from build123d import *

# Parameters (mm, degrees)
F0_R     = 10
F1_DEPTH = 50
F0_W     = 50
F0_H     = 15
F2_DEPTH = 15
F3_W     = 50
F3_H     = 15
F4_DEPTH = 35
F6_DEPTH = 27.501
F8_DEPTH = 257.5


with BuildPart() as f1:
    # F0 (on Front) → F1 (new body)
    with BuildSketch(Plane.XZ):
        with BuildLine():
            ThreePointArc((18.540496, 7.5), (13.624005, 14.641943), (6.146908, 19.03196))
            ThreePointArc((6.146908, 19.03196), (-18.120519, -8.464442), (18.540496, -7.5))
            ThreePointArc((18.540496, -7.5), (19.631734, -3.820345), (20, 0))
            ThreePointArc((20, 0), (19.631734, 3.820345), (18.540496, 7.5))
        make_face()
        Circle(F0_R, mode=Mode.SUBTRACT)
        with BuildLine():
            Line((27.149505, -7.5), (27.149505, 7.5))
            Line((27.149505, 7.5), (18.540496, 7.5))
            ThreePointArc((18.540496, 7.5), (19.631734, 3.820345), (20, 0))
            ThreePointArc((20, 0), (19.631734, -3.820345), (18.540496, -7.5))
            Line((18.540496, -7.5), (27.149505, -7.5))
        make_face()
    extrude(amount=F1_DEPTH)

    # F0 (on Front) → F2 (join)
    with BuildSketch(Plane.XZ):
        with BuildLine():
            Line((77.149505, 7.5), (77.149505, 24.5))
            ThreePointArc((77.149505, 24.5), (61.595967, 43.999461), (39.126608, 33.170362))
            ThreePointArc((39.126608, 33.170362), (25.287149, 19.918772), (6.146908, 19.03196))
            ThreePointArc((6.146908, 19.03196), (13.624005, 14.641943), (18.540496, 7.5))
            Line((18.540496, 7.5), (27.149505, 7.5))
            Line((27.149505, 7.5), (77.149505, 7.5))
        make_face()
        with Locations((57.149505, 24.5)):
            Circle(F0_R, mode=Mode.SUBTRACT)
        with Locations((52.149505, 0)):
            Rectangle(F0_W, F0_H)
    extrude(amount=F2_DEPTH)

    # F3 (on face) → F4 (join)
    with BuildSketch(Plane.XZ.offset(15)):
        with Locations((52.149505, 0)):
            Rectangle(F3_W, F3_H)
    extrude(amount=F4_DEPTH)

    # F5 (on face) → F6 (join, through all)
    with BuildSketch(Plane.XY.offset(7.5)):
        Polygon((77.149505, -25), (27.149505, -50), (77.149505, -50), align=None)
    extrude(amount=-F6_DEPTH)

    # F7 (on face) → F8 (cut)
    with BuildSketch(Plane.XY.offset(7.5)):
        Polygon((77.149505, -25), (27.149505, -50), (77.149505, -50), align=None)
    extrude(amount=-F8_DEPTH, mode=Mode.SUBTRACT)


solid = f1.part
Can you work these out from the model? Positions are in its coordinate system, mm. A direction names the side the tool comes from. Coordinates: 2 decimals unless noted, no trailing zeros. Write each loop counter-clockwise with the first axis right and the second up, starting at its lowest first coordinate (ties: lowest second). Pieces come first, ordered by that corner, then holes. Notation, with made-up numbers: (3, -18.75) - (62, -18.75) arc R22 cw to (62, 16.25) - close; hole circle Ø8 at (-25, 31). An arc over 180 degrees is marked (long way). Return JSON: item names as keys, results as strings. Group by question number.
Item 1: I'm going to push flat-ended pins straight in: pin 1 Ø6 at (x, y) = (5.5, -26.5) entering from -Z; pin 2 Ø2 at (y, z) = (-17.5, 9) entering from +X; pin 3 Ø15 at (x, y) = (42, -23.5) entering from -Z. Where does each tip first touch, or does it pass through?
Item 2: We'd pull the mould along X, two halves only. Please class faces 4 (the face through (25.54, -7.4, 20.03)), 5 (the face through (8, -50, 9)), 6 (the face through (52.5, -37.325, 0.105)): pulls with the +X half, pulls with the -X half, needs draft (parallel to the pull), parting line crosses it, or undercut.
Item 3: If we section it at B-B (x = 0): Write out the boundary of the cut face in (y, z).
Item 4: Which directions (+Z, -Z, +X, -X, +Y, -Y) give clear straight access to the entire face, cutting with the end or side of a thin tool? Please do faces 1 (the face through (41, -19, -7.5)), 2 (the face through (49, -15, 18)), 3 (the face through (61.963, -7.395, 43.912)).
Item 5: If we section it at A-A (y = -13): Write out the boundary of the cut face in (x, z), then the cut area to 3 significant figures.
Item 6: If we section it at C-C (z = 0): Write out the boundary of the cut face in (x, y).
Item 7: If we section it at D-D (y = -18): Write out the boundary of the cut face in (x, z), then the cut area to 3 significant figures.
Item 8: Please list where these lines run through material, in increasing order: probe 1 along Z at (x, y) = (0, -19); probe 2 along Y at (x, z) = (50.5, 40); probe 3 along Z at (x, y) = (23.5, -24).
Return value:
{
 "1": {"pin 1": "stops at z = -19.84", "pin 2": "stops at x = 18.33", "pin 3": "stops at z = -7.5"},
 "2": {"face 4": "undercut", "face 5": "needs draft", "face 6": "pulls with the +X half"},
 "3": {"outline": "(-50, -20) - (0, -20) - (0, -10) - (-50, -10) - close; (-50, 10) - (0, 10) - (0, 20) - (-50, 20) - close"},
 "4": {"face 1": "-Z, +X, +Y, -Y", "face 2": "+Z, +X, -Y", "face 3": "+Z, +Y, -Y"},
 "5": {"outline": "(6.15, 19.03) arc R20 ccw (long way) to (18.54, -7.5) - (77.15, -7.5) - (77.15, 24.5) arc R20 ccw to (39.13, 33.17) arc R27.29 cw to start; hole circle Ø20 at (0, 0); hole circle Ø20 at (57.15, 24.5)", "area": "3,110 mm^2"},
 "6": {"outline": "(-20, -50) - (-10, -50) - (-10, 0) - (-20, 0) - close; (10, -50) - (27.15, -50) - (77.15, -25) - (77.15, 0) - (10, 0) - close"},
 "7": {"outline": "(6.15, 19.03) arc R20 ccw (long way) to (18.54, -7.5) - (77.15, -7.5) - (77.15, 7.5) - (18.54, 7.5) arc R20 ccw to start; hole circle Ø20 at (0, 0)", "area": "1,810 mm^2"},
 "8": {"probe 1": "z = -20 to -10, 10 to 20", "probe 2": "y = -15 to 0", "probe 3": "z = -7.5 to 7.5"}
}
